from build123d import *

# Parameters (mm, degrees)
F0_R     = 6
F1_DEPTH = 25
F2_W     = 35
F2_H     = 10
F3_DEPTH = 20.501
F5_DEPTH = 12.5
F6_R     = 5
F7_R     = 5
F8_DEPTH = 15


with BuildPart() as f1:
    # F0 (on Front) → F1 (new body)
    with BuildSketch(Plane.XZ):
        with BuildLine():
            ThreePointArc((9.604686, -8), (11.753905, -4.253905), (12.5, 0))
            ThreePointArc((12.5, 0), (11.753905, 4.253905), (9.604686, 8))
            ThreePointArc((9.604686, 8), (-12.5, 0), (9.604686, -8))
        make_face()
        Circle(F0_R, mode=Mode.SUBTRACT)
        with BuildLine():
            ThreePointArc((9.604686, 8), (11.753905, 4.253905), (12.5, 0))
            ThreePointArc((12.5, 0), (11.753905, -4.253905), (9.604686, -8))
            Line((9.604686, -8), (79, -8))
            ThreePointArc((79, -8), (75, 0), (79, 8))
            Line((79, 8), (9.604686, 8))
        make_face()
        with BuildLine():
            ThreePointArc((95, 0), (89.472136, 8.944272), (79, 8))
            ThreePointArc((79, 8), (75, 0), (79, -8))
            ThreePointArc((79, -8), (89.472136, -8.944272), (95, 0))
        make_face()
        with Locations((85, 0)):
            Circle(F0_R, mode=Mode.SUBTRACT)
    extrude(amount=F1_DEPTH)

    # F2 (on face) → F3 (cut, through all)
    with BuildSketch(Plane.XY.offset(8)):
        with Locations((27.104686, -5)):
            Rectangle(F2_W, F2_H)
    extrude(amount=-F3_DEPTH, mode=Mode.SUBTRACT)

    # F4 (on face) → F5 (cut, symmetric)
    with BuildSketch(Plane.YZ.offset(9.604686)):
        Polygon((0, 8), (-10, 8), (0, -8), align=None)
    extrude(amount=F5_DEPTH, both=True, mode=Mode.SUBTRACT)

    # F6
    f6_edges = [f1.edges().sort_by_distance(p)[0] for p in [
        (44.604686, -10, 0),
    ]]
    fillet(f6_edges, radius=F6_R)

    # F7 (on face) → F8 (join)
    with BuildSketch(Plane(origin=(0, 0, -8), x_dir=(1, 0, 0), z_dir=(0, 0, -1))):
        with Locations((64, 12.5)):
            Circle(F7_R)
    extrude(amount=F8_DEPTH)


solid = f1.part
Verification items for the finished model (mm, model axes). A direction names the side the tool comes from. Round coordinates to 2 decimals unless told otherwise and drop trailing zeros. Write each loop counter-clockwise with the first axis right and the second up, starting at its lowest first coordinate (ties: lowest second). Pieces come first, ordered by that corner, then holes.
(1) Mould release check, pull along X, two halves, no side actions. Record for faces 5 (the flat face through (-7, 0, 0)), 6 (the flat face through (6.22, -5.07, 0.11)): pulls with the +X half, pulls with the -X half, needs draft (parallel to the pull), parting line crosses it, or undercut.
Returned:
face 5: needs draft
face 6: undercut
(2) Access from +Z, -Z, +X, -X, +Y, -Y to the whole of each face (thin tool, end or side, straight path). Record for faces 1 (the cylindrical face through (63.349, -17.457, -15.395)), 2 (the flat face through (3, -5, 8)), 3 (the flat face through (52, -15, 8)), 4 (the flat face through (9.605, -7, -3)).
Returned:
face 1: -Z
face 2: +Y
face 3: +Z, +Y, -Y
face 4: +Z, -Z, +Y
(3) Depth check by flat-ended pin: pin 1 Ø1 at (x, y) = (52.5, -21) entering from -Z; pin 2 Ø0.8 at (y, z) = (-6.5, 6.5) entering from +X; pin 3 Ø6 at (y, z) = (-5.5, 4.5) entering from +X. Enter the tip coordinate at first touch or a pass-through.
Returned:
pin 1: stops at z = -8
pin 2: stops at x = 92.92
pin 3: stops at x = 94.89
(4) Material ranges on line 1 (X direction, y = -1.5, z = -5); line 2 (Z direction, x = 85, y = -8); line 3 (Z direction, x = 0, y = -12), recorded low to high.
Returned:
line 1: x = -11.46 to -3.32, 44.6 to 81.68, 88.32 to 93.66
line 2: z = -10 to -6, 6 to 10
line 3: z = -12.5 to -6, 6 to 12.5
(5) Section check D-D (z = -9). Enter the section's corners in (x, y).
Returned:
outline: (-8.67, -25) - (8.67, -25) - (8.67, 0) - (-8.67, 0) - close; circle Ø10 at (64, -12.5); (80.64, -25) - (89.36, -25) - (89.36, 0) - (80.64, 0) - close
(6) Section check C-C (y = -6). Enter the section's corners in (x, z).
Returned:
outline: (-2.9, 5.26) - (-2.9, 8) - (9.6, 8) arc R12.5 ccw (long way) to (9.6, -8) - (9.6, 1.6) - (5.78, 1.6) arc R6 cw (long way) to start; (44.5, -8) - (79, -8) arc R10 ccw (long way) to (79, 8) - (44.5, 8) - close; hole circle Ø12 at (85, 0)
(7) Section check A-A (y = -12.5). Enter the section's corners in (x, z), plus the area to 3 significant figures.
Returned:
outline: (9.6, -8) - (59, -8) - (59, -23) - (69, -23) - (69, -8) - (79, -8) arc R10 ccw (long way) to (79, 8) - (9.6, 8) arc R12.5 ccw (long way) to start; hole circle Ø12 at (0, 0); hole circle Ø12 at (85, 0)
area: 1,760 mm2
(8) Section check B-B (x = 0). Enter the section's corners in (y, z), plus the area to 3 significant figures.
Returned:
outline: (-25, -12.5) - (0, -12.5) - (0, -8) - (-1.25, -6) - (-25, -6) - close; (-25, 6) - (-8.75, 6) - (-10, 8) - (0, 8) - (0, 12.5) - (-25, 12.5) - close
area: 305 mm2
